```python
from build123d import *

# Parameters (mm, degrees)
F1_W     = 48.65
F1_H     = 48.65
F2_DEPTH = 3.175
F3_W     = 3.175
F3_H     = 15
F3_W_2   = 15
F3_H_2   = 3.175
F4_DEPTH = 3.175


with BuildPart() as f2:
    # F1 (on Top) → F2 (new body)
    with BuildSketch(Plane.XY):
        Rectangle(F1_W, F1_H)
    extrude(amount=F2_DEPTH)

    # F3 (on face) → F4 (join, through all)
    with BuildSketch(Plane.XY.offset(3.175)):
        with Locations((-25.9125, 0)):
            Rectangle(F3_W, F3_H)
        with Locations((0, 25.9125)):
            Rectangle(F3_W_2, F3_H_2)
        with Locations((0, -25.9125)):
            Rectangle(F3_W_2, F3_H_2)
        with Locations((25.9125, 0)):
            Rectangle(F3_W, F3_H)
    extrude(amount=-F4_DEPTH)


solid = f2.part
```
Input: part model. Units: mm. Frame: model coordinates. A direction names the side the tool comes from. Round coordinates to 2 decimals unless told otherwise and drop trailing zeros. Write each loop counter-clockwise with the first axis right and the second up, starting at its lowest first coordinate (ties: lowest second). Pieces come first, ordered by that corner, then holes. Notation, with made-up numbers: (1, 76.25) -> (51, 76.25) arc R12 cw to (51, 87.25) -> close; hole circle Ø4 at (9.5, 28.5). An arc over 180 degrees is marked (long way). Answer as CSV lines item,"result".
1. Reachability of faces 1 (the flat face through (7.5, -26, 2)), 2 (the flat face through (-24.325, -16, 2)), 3 (the flat face through (-26, 7.5, 2)) from +Z, -Z, +X, -X, +Y, -Y: full face, straight path, thin tool, end or side. Return the list, or none.
Geometry says:
face 1,"+Z, -Z, +X, -Y"
face 2,"+Z, -Z, -X, -Y"
face 3,"+Z, -Z, -X, +Y"
2. Contact query for flat-ended pins moving along their axis: P1, Ø1.6, axis at x = -25.5, z = 2, coming from the -Y side; P2, Ø1.6, axis at y = -25.5, z = 1.5, coming from the -X side; P3, Ø4, axis at x = 21, y = -15.5, coming from the -Z side; P4, Ø1.6, axis at y = 13.5, z = 1.5, coming from the +X side (3 decimals). Output: stop coordinate, or through.
Geometry says:
P1,"stops at y = -7.5"
P2,"stops at x = -7.5"
P3,"stops at z = 0"
P4,"stops at x = 24.325"
3. Ray query, L1, parallel to X at y = -21.5, z = 1.2 (3 decimals); L2, parallel to X at y = 25, z = 0.95. Return the intervals inside material, ascending. Write a range as [from, to].
Geometry says:
L1,"x = [-24.325, 24.325]"
L2,"x = [-7.5, 7.5]"
4. Section B-B (y = 15.5). Return the cut outline in (x, z) (3 decimals).
Geometry says:
outline,"(-24.325, 0) -> (24.325, 0) -> (24.325, 3.175) -> (-24.325, 3.175) -> close"
5. Section A-A (z = 2). Return the cut outline in (x, y) (3 decimals), plus the area to 3 significant figures.
Geometry says:
outline,"(-27.5, -7.5) -> (-24.325, -7.5) -> (-24.325, -24.325) -> (-7.5, -24.325) -> (-7.5, -27.5) -> (7.5, -27.5) -> (7.5, -24.325) -> (24.325, -24.325) -> (24.325, -7.5) -> (27.5, -7.5) -> (27.5, 7.5) -> (24.325, 7.5) -> (24.325, 24.325) -> (7.5, 24.325) -> (7.5, 27.5) -> (-7.5, 27.5) -> (-7.5, 24.325) -> (-24.325, 24.325) -> (-24.325, 7.5) -> (-27.5, 7.5) -> close"
area,"2,560 mm^2"
